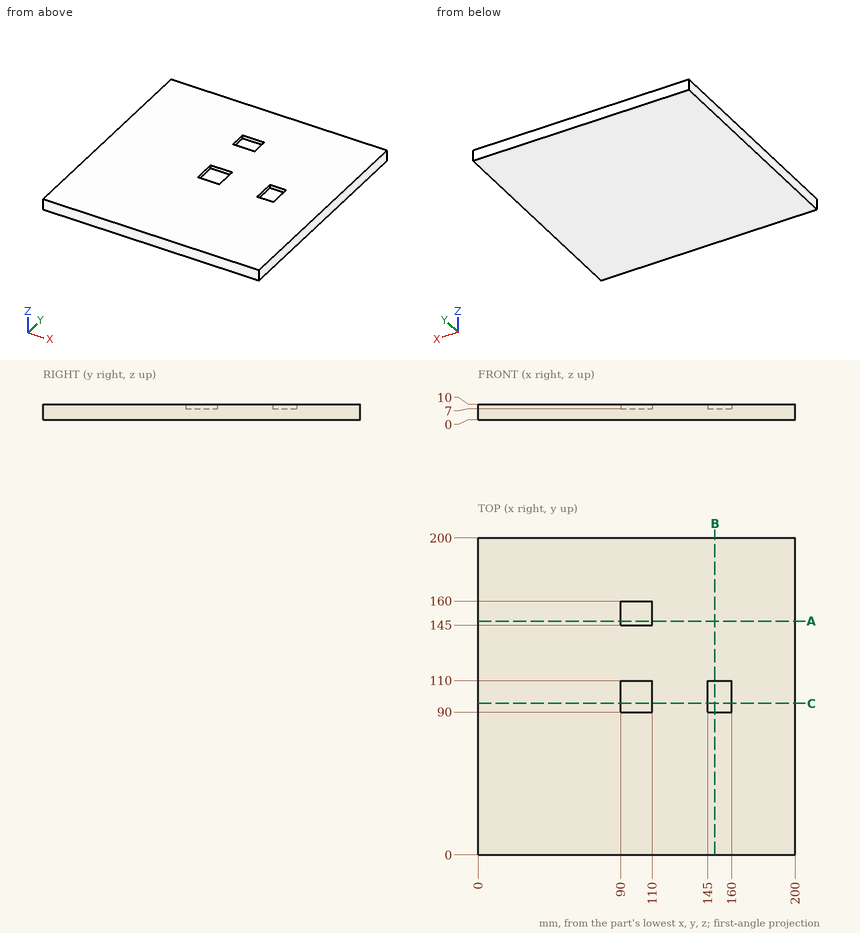
Part print with two shaded views. Sizes in mm from the minimum x, y, z corner. Give positions to 0.01 mm unless a question says otherwise; leave off trailing zeros. Order: outer loops, then holes, each group sorted by start corner. A loop starts at its lowest first (then second) coordinate and runs counter-clockwise, first axis right, second up. Notation, with made-up numbers: M -28,24.25 L -11,24.25 A24 cw -11,37.25 Z; hole C 77.5,-10 d9. An arc over 180 degrees is marked long. Write item = value, one per line.
Q1. Drill centre line: line 1 (X direction, y = 153.5, z = 9). Where is it in solid material? Low to high. Write a range as [from, to].
Derived:
line_1 = [0, 90], [110, 200]
Q2. Cut at C-C, the plane y = 95.5. List the corners of the cut face in (x, z), then the cut area to 4 significant figures.
Derived:
outline = M 0,0 L 200,0 L 200,10 L 160,10 L 160,7 L 145,7 L 145,10 L 110,10 L 110,7 L 90,7 L 90,10 L 0,10 Z
area = 1,895 mm2
Q3. Cut at A-A, the plane y = 147.5. List the corners of the cut face in (x, z), then the cut area to 3 significant figures.
Derived:
outline = M 0,0 L 200,0 L 200,10 L 110,10 L 110,7 L 90,7 L 90,10 L 0,10 Z
area = 1,940 mm2
Q4. Flat gauge pin, fed straight in: pin 1 (4.5 mm diameter, centred on x = 156, y = 97.5, fed in from +Z). Where does the tip first touch, or does it go through?
Derived:
pin_1 = 7
